Input: part model. Units: mm. Frame: model coordinates. A direction names the side the tool comes from. Coordinates: 2 decimals unless noted, no trailing zeros. Loops run counter-clockwise (first coordinate to the right, second up) from the corner with the lowest first, then second, coordinate; pieces in that order, holes last.
(1) Set-up query: faces 1 (the face through (-37, 0, 280)), 2 (the face through (32, 0, 250)), 3 (the face through (-33, 0, 250)). Return all of +Z, -Z, +X, -X, +Y, -Y with unobstructed straight access to the full face (end or side cutting, diameter ignored); none if empty.
(2) Line query: L1, parallel to X at y = 15, z = 263; L2, parallel to X at y = -9, z = 154; L3, parallel to Z at x = 7, y = -10.5. Output: solid intervals per line, ascending.
(3) Contact query for flat-ended pins moving along their axis: P1, Ø15, axis at y = -11, z = 124.5, coming from the +X side; P2, Ø4, axis at x = 35, y = -0.5, coming from the -Z side; P3, Ø25, axis at y = 0.5, z = 133, coming from the -X side. Output: stop coordinate, or through.
(4) Section C-C, the plane x = -33.5. Return loops of the section in (y, z).
(5) Section B-B, the plane z = 55. Return loops of the section in (x, y), then the cut area to 3 significant figures.
(6) Section A-A, the plane y = 19.5. Return loops of the section in (x, z), then the cut area to 3 significant figures.
```python
from build123d import *

# Parameters (mm, degrees)
SZKIC1_W                    = 40
SZKIC1_H                    = 50
DODANIE_WYCI_GNI_CIE1_DEPTH = 250
SZKIC2_W                    = 90
SZKIC2_H                    = 50
DODANIE_WYCI_GNI_CIE2_DEPTH = 10
SZKIC3_W                    = 8
SZKIC3_H                    = 50
DODANIE_WYCI_GNI_CIE3_DEPTH = 40


with BuildPart() as part:
    # Szkic1 → Dodanie-wyciągnięcie1 (new body)
    with BuildSketch(Plane.XY):
        Rectangle(SZKIC1_W, SZKIC1_H)
    extrude(amount=DODANIE_WYCI_GNI_CIE1_DEPTH)

    # Szkic2 → Dodanie-wyciągnięcie2 (add)
    with BuildSketch(Plane.XY.offset(250)):
        Rectangle(SZKIC2_W, SZKIC2_H)
    extrude(amount=DODANIE_WYCI_GNI_CIE2_DEPTH)

    # Szkic3 → Dodanie-wyciągnięcie3 (add)
    with BuildSketch(Plane.XY.offset(260)):
        with Locations((-41, 0)):
            Rectangle(SZKIC3_W, SZKIC3_H)
        with Locations((41, 0)):
            Rectangle(SZKIC3_W, SZKIC3_H)
    extrude(amount=DODANIE_WYCI_GNI_CIE3_DEPTH)


solid = part.part
```
Report:
1. face 1: +Z, +Y, -Y
1. face 2: -Z, +X, +Y, -Y
1. face 3: -Z, -X, +Y, -Y
2. L1: x = -45 to -37, 37 to 45
2. L2: x = -20 to 20
2. L3: z = 0 to 260
3. P1: stops at x = 20
3. P2: stops at z = 250
3. P3: stops at x = -20
4. outline: (-25, 250) - (25, 250) - (25, 260) - (-25, 260) - close
5. outline: (-20, -25) - (20, -25) - (20, 25) - (-20, 25) - close
5. area: 2,000 mm2
6. outline: (-45, 250) - (-20, 250) - (-20, 0) - (20, 0) - (20, 250) - (45, 250) - (45, 300) - (37, 300) - (37, 260) - (-37, 260) - (-37, 300) - (-45, 300) - close
6. area: 11,500 mm2
